The figure shows three views and two pictorial views of one solid part (mm, origin at its lowest corner). Answer the questions. Coordinates: 2 decimals unless noted, no trailing zeros. Order: outer loops, then holes, each group sorted by start corner. A loop starts at its lowest first (then second) coordinate and runs counter-clockwise, first axis right, second up. Notation, with made-up numbers: (-3, 79.25) -> (55, 79.25) arc R26 cw to (55, 101.25) -> close; hole circle Ø9 at (80, 62.5). An arc over 180 degrees is marked (long way). Use one line per item in the form item = value.
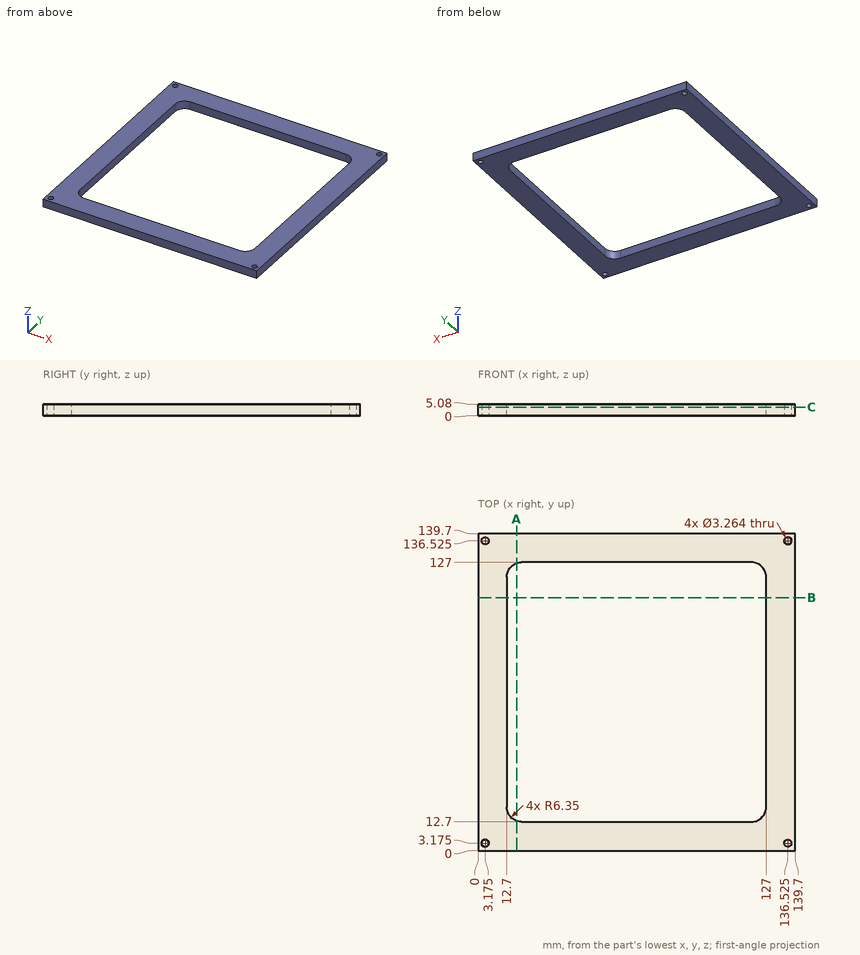
(1) Section A-A on x = 17 is taken. Write down the section's boundary in (y, z).
Data:
outline = (0, 0) -> (13.04, 0) -> (13.04, 5.08) -> (0, 5.08) -> close; (126.66, 0) -> (139.7, 0) -> (139.7, 5.08) -> (126.66, 5.08) -> close
(2) Straight lines are drawn through the part: line 1 along Y through (x, z) = (24, 1.4); line 2 along X through (y, z) = (16.5, 2.3). For each, find the intervals that lie inside material, in ascending order.
Data:
line_1 = 0 to 12.7, 127 to 139.7
line_2 = 0 to 13.23, 126.47 to 139.7
(3) Section B-B on y = 111.5 is taken. Write down the section's boundary in (x, z).
Data:
outline = (0, 0) -> (12.7, 0) -> (12.7, 5.08) -> (0, 5.08) -> close; (127, 0) -> (139.7, 0) -> (139.7, 5.08) -> (127, 5.08) -> close
(4) Section C-C on z = 3.7 is taken. Write down the section's boundary in (x, y) (3 decimals), plus the area to 3 significant figures.
Data:
outline = (0, 0) -> (139.7, 0) -> (139.7, 139.7) -> (0, 139.7) -> close; hole circle Ø3.264 at (3.175, 3.175); hole circle Ø3.264 at (3.175, 136.525); hole (12.7, 19.05) arc R6.35 ccw to (19.05, 12.7) -> (120.65, 12.7) arc R6.35 ccw to (127, 19.05) -> (127, 120.65) arc R6.35 ccw to (120.65, 127) -> (19.05, 127) arc R6.35 ccw to (12.7, 120.65) -> close; hole circle Ø3.264 at (136.525, 3.175); hole circle Ø3.264 at (136.525, 136.525)
area = 6,450 mm²
(5) This flat-tipped pin is pushed along its axis until it touches: P1, Ø2.5, axis at x = 136.525, y = 3.175, coming from the +Z side. Where does it stop, or does it pass through?
Data:
P1 = through
